Build history of the part. All positions in model axes, mm. Face numbers are marked on the shaded views. A direction names the side the tool comes from. Round coordinates to 2 decimals unless told otherwise and drop trailing zeros. Loops run counter-clockwise (first coordinate to the right, second up) from the corner with the lowest first, then second, coordinate; pieces in that order, holes last. Notation, with made-up numbers: (50.5, 43) - (107.5, 43) arc R10 cw to (107.5, 60) - close; hole circle Ø2 at (53.25, -40). An arc over 180 degrees is marked (long way). Use a Markdown table: item, result.
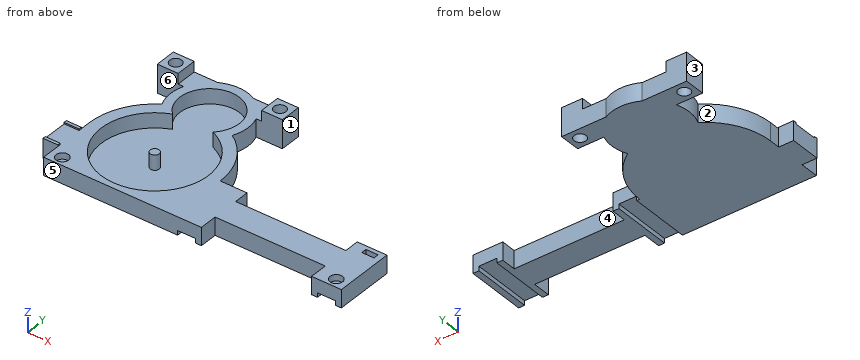
from build123d import *

# Parameters (mm, degrees)
SKETCH016_R     = 2
PAD012_DEPTH    = 6
SKETCH001_R     = 1.5
POCKET_DEPTH    = 5
SKETCH010_W     = 6
SKETCH010_H     = 1.5
POCKET009_DEPTH = 20
SKETCH017_R     = 2.1
SKETCH017_W     = 4.1
SKETCH017_H     = 1.8
POCKET010_DEPTH = 2.1
PAD013_DEPTH    = 5
SKETCH_W        = 7
SKETCH_H        = 7
SKETCH_R        = 2
PAD014_DEPTH    = 3.5
SKETCH020_R     = 2.1
SKETCH020_W     = 4.1
SKETCH020_H     = 1.8
POCKET017_DEPTH = 2.1


with BuildPart() as part:
    # Sketch016 → Pad012 (new body)
    with BuildSketch(Plane.XY):
        with BuildLine():
            Line((0, 0), (0, 20))
            ThreePointArc((10.1918, 38.5625), (2.715545, 30.588192), (0, 20))
            ThreePointArc((9.803689, 48.5), (9.009903, 43.49267), (10.1918, 38.5625))
            Line((9.803689, 48.5), (1, 48.5))
            Line((1, 48.5), (1, 55.5))
            Line((1, 55.5), (15.937822, 55.5))
            ThreePointArc((28.062178, 55.5), (22, 57), (15.937822, 55.5))
            Line((43, 55.5), (28.062178, 55.5))
            Line((43, 55.5), (43, 48.5))
            Line((34.196311, 48.5), (43, 48.5))
            ThreePointArc((33.8082, 38.5625), (34.990097, 43.49267), (34.196311, 48.5))
            ThreePointArc((44, 20), (41.284455, 30.588191), (33.8082, 38.5625))
            Line((53, 20), (44, 20))
            Line((53, 15), (53, 20))
            Line((90, 15), (53, 15))
            Line((90, 20), (90, 15))
            Line((100, 20), (90, 20))
            Line((100, 0), (100, 20))
            Line((90, 0), (100, 0))
            Line((90, 6), (90, 0))
            Line((53, 6), (90, 6))
            Line((53, 0), (53, 6))
            Line((0, 0), (53, 0))
        make_face()
        with Locations((4.5, 52)):
            Circle(SKETCH016_R, mode=Mode.SUBTRACT)
        with Locations((39.5, 52)):
            Circle(SKETCH016_R, mode=Mode.SUBTRACT)
    extrude(amount=PAD012_DEPTH)

    # Sketch001 → Pocket (cut)
    with BuildSketch(Plane.XY.offset(6)):
        with BuildLine():
            ThreePointArc((28.798693, 36.666667), (22, 54), (15.201307, 36.666667))
            ThreePointArc((15.201307, 36.666667), (22, 2), (28.798693, 36.666667))
        make_face()
        with Locations((22, 20)):
            Circle(SKETCH001_R, mode=Mode.SUBTRACT)
    extrude(amount=-POCKET_DEPTH, mode=Mode.SUBTRACT)

    # Sketch010 → Pocket009 (cut)
    with BuildSketch(Plane.XZ):
        with Locations((48, 0.75)):
            Rectangle(SKETCH010_W, SKETCH010_H)
        with Locations((95, 0.75)):
            Rectangle(SKETCH010_W, SKETCH010_H)
    extrude(amount=-POCKET009_DEPTH, mode=Mode.SUBTRACT)

    # Sketch017 → Pocket010 (cut)
    with BuildSketch(Plane(origin=(0, 0, 0), x_dir=(1, 0, 0), z_dir=(0, 0, -1))):
        with Locations((4, 3)):
            Circle(SKETCH017_R)
        with Locations((96, 3)):
            Circle(SKETCH017_R)
        with Locations((96, 17.75)):
            Rectangle(SKETCH017_W, SKETCH017_H)
    extrude(amount=-POCKET010_DEPTH, mode=Mode.SUBTRACT)

    # Sketch015 → Pad013 (new body)
    with BuildSketch(Plane(origin=(0, 0, 0), x_dir=(0, -1, 0), z_dir=(-1, 0, 0))):
        Polygon((-16.5, 6.5), (-16.5, 0), (-6.25, 0), (-6.25, 6.5), (-7.25, 6.5), (-7.25, 6), (-15.5, 6), (-15.5, 6.5), align=None)
    extrude(amount=PAD013_DEPTH)

    # Sketch → Pad014 (new body)
    with BuildSketch(Plane.XY.offset(6)):
        with Locations((4.5, 52)):
            Rectangle(SKETCH_W, SKETCH_H)
        with Locations((4.5, 52)):
            Circle(SKETCH_R, mode=Mode.SUBTRACT)
        with Locations((39.5, 52)):
            Rectangle(SKETCH_W, SKETCH_H)
        with Locations((39.5, 52)):
            Circle(SKETCH_R, mode=Mode.SUBTRACT)
    extrude(amount=PAD014_DEPTH)

    # Sketch020 → Pocket017 (cut)
    with BuildSketch(Plane.XY.offset(6)):
        with Locations((4, 3)):
            Circle(SKETCH020_R)
        with Locations((96, 3)):
            Circle(SKETCH020_R)
        with Locations((96, 17.75)):
            Rectangle(SKETCH020_W, SKETCH020_H)
    extrude(amount=-POCKET017_DEPTH, mode=Mode.SUBTRACT)


solid = part.part
Q1. Cut at A-A, the plane y = 52. List the corners of the cut face in (x, z), plus the area to 3 significant figures.
Results found:
| item | result |
|---|---|
| outline | (1, 0) - (2.5, 0) - (2.5, 9.5) - (1, 9.5) - close; (6.5, 0) - (37.5, 0) - (37.5, 9.5) - (36, 9.5) - (36, 6) - (28, 6) - (28, 1) - (16, 1) - (16, 6) - (8, 6) - (8, 9.5) - (6.5, 9.5) - close; (41.5, 0) - (43, 0) - (43, 9.5) - (41.5, 9.5) - close |
| area | 165 mm2 |
Q2. Which spindle directions (+Z, -Z, +X, -X, +Y, -Y) get a long thin tool onto all of the face, cutting with end or side? Do the marked faces 1, 2 and 3. Say none if no direction does.
Results found:
| item | result |
|---|---|
| face 1 | +Z, -Z, +X, +Y |
| face 2 | +Z, -Z, -X |
| face 3 | +Z, -Z, -X, +Y |
Q3. Cut at D-D, the plane y = 3. List the corners of the cut face in (x, z), plus the area to 3 significant figures.
Results found:
| item | result |
|---|---|
| outline | (0, 0) - (45, 0) - (45, 1.5) - (51, 1.5) - (51, 0) - (53, 0) - (53, 6) - (27.92, 6) - (27.92, 1) - (16.08, 1) - (16.08, 6) - (6.1, 6) - (6.1, 3.9) - (1.9, 3.9) - (1.9, 6) - (0, 6) - close; (90, 0) - (92, 0) - (92, 1.5) - (98, 1.5) - (98, 0) - (100, 0) - (100, 6) - (98.1, 6) - (98.1, 3.9) - (93.9, 3.9) - (93.9, 6) - (90, 6) - close |
| area | 283 mm2 |
Q4. Probe line 1 (X direction, y = 44, z = 3.5); line 2 (Y direction, x = 36.5, z = 3.75); line 3 (X direction, y = 10, z = 5.5). List the from-to ranges inside material, lowest first.
Results found:
| item | result |
|---|---|
| line 1 | x = 9 to 12, 32 to 35 |
| line 2 | y = 0 to 9.33, 30.67 to 36.55, 48.5 to 55.5 |
| line 3 | x = -5 to 7.03, 36.97 to 100 |
Q5. Cut at C-C, the plane x = 96. List the corners of the cut face in (y, z), plus the area to 3 significant figures.
Results found:
| item | result |
|---|---|
| outline | (0, 1.5) - (20, 1.5) - (20, 6) - (18.65, 6) - (18.65, 3.9) - (16.85, 3.9) - (16.85, 6) - (5.1, 6) - (5.1, 3.9) - (0.9, 3.9) - (0.9, 6) - (0, 6) - close |
| area | 77.4 mm2 |
Q6. Cut at B-B, the plane z = 8. List the corners of the cut face in (x, y), plus the area to 3 significant figures.
Results found:
| item | result |
|---|---|
| outline | (1, 48.5) - (8, 48.5) - (8, 55.5) - (1, 55.5) - close; (36, 48.5) - (43, 48.5) - (43, 55.5) - (36, 55.5) - close; hole circle Ø4 at (4.5, 52); hole circle Ø4 at (39.5, 52) |
| area | 72.9 mm2 |
Q7. Pull direction Y, two halves, no side cores. Call the marked faces 4, 5 and 6: pulls with the +Y half, pulls with the -Y half, needs draft (parallel to the pull), parting line crosses it, or undercut.
Results found:
| item | result |
|---|---|
| face 4 | pulls with the +Y half |
| face 5 | pulls with the -Y half |
| face 6 | undercut |
Q8. Drop flat-ended pins along their axis: pin 1 (3.5 mm diameter, centred on y = 53, z = 6, fed in from -X); pin 2 (5 mm diameter, centred on y = 3.5, z = 2.5, fed in from -X); pin 3 (1.3 mm diameter, centred on x = 95.5, y = 2.5, fed in from +Z). Give the stop position or say it passes through.
Results found:
| item | result |
|---|---|
| pin 1 | stops at x = 1 |
| pin 2 | stops at x = 0 |
| pin 3 | stops at z = 3.9 |
